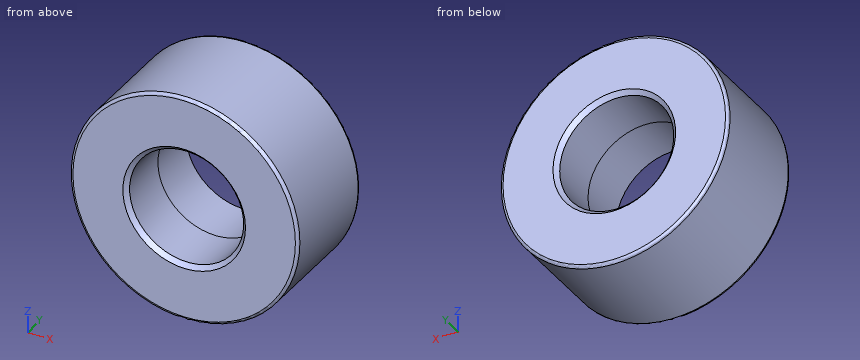
from build123d import *

# Parameters (mm, degrees)
SKETCH1_R                = 4
SKETCH1_R_2              = 2
BOSS_EXTRUDE1_DEPTH      = 1.875
BOSS_EXTRUDE1_DEPTH_BACK = 1.875
FILLET1_R                = 0.1
CHAMFER4_SIZE            = 0.15


with BuildPart() as part:
    # Sketch1 → Boss-Extrude1 (new body, two sides)
    with BuildSketch(Plane(origin=(0, 0, 0), x_dir=(1, 0, 0), z_dir=(0, 1, 0))) as boss_extrude1_sk:
        Circle(SKETCH1_R)
        Circle(SKETCH1_R_2, mode=Mode.SUBTRACT)
    extrude(amount=BOSS_EXTRUDE1_DEPTH)
    extrude(boss_extrude1_sk.sketch, amount=-BOSS_EXTRUDE1_DEPTH_BACK)

    # Fillet1
    fillet1_edges = [part.edges().sort_by_distance(p)[0] for p in [
        (-4, -1.875, 0),
        (-4, 1.875, 0),
    ]]
    fillet(fillet1_edges, radius=FILLET1_R)

    # Chamfer4
    chamfer4_edges = [part.edges().sort_by_distance(p)[0] for p in [
        (-2, -1.875, 0),
        (-2, 1.875, 0),
    ]]
    chamfer(chamfer4_edges, length=CHAMFER4_SIZE)


solid = part.part
Design review of the part built by this model. Coordinates are the model's own, in mm. Give positions to 0.01 mm unless a question says otherwise; leave off trailing zeros. Write each loop counter-clockwise with the first axis right and the second up, starting at its lowest first coordinate (ties: lowest second). Pieces come first, ordered by that corner, then holes. Notation, with made-up numbers: M 32,48.25 L 40,48.25 A7 cw 40,52.25 Z; hole C -15.75,-7 d9. An arc over 180 degrees is marked long. Return JSON: item names as keys, results as strings. Group by question number.
Item 1: Clearance check with a flat-ended pin moving along its axis: pin 1 Ø1.5 at (x, y) = (2.5, -1) entering from -Z. State where the tip first meets the part, or that it passes through.
Item 2: Wall thickness on line 1 along Z through (x, y) = (0, -0.8); line 2 along X through (y, z) = (-1.2, -0.75): over which ranges is each line inside the solid? List them lowest first.
Item 3: Take a section at A-A (x = 0). Give the boundary of the cut face in (y, z) (3 decimals), plus the area to 3 significant figures.
Item 4: Take a section at B-B (z = 0). Give the boundary of the cut face in (x, y) (3 decimals).
Item 5: Take a section at C-C (y = -0.3). Give the boundary of the cut face in (x, z).
Return value:
{
 "1": {"pin 1": "stops at z = -3.6"},
 "2": {"line 1": "z = -4 to -2, 2 to 4", "line 2": "x = -3.93 to -1.85, 1.85 to 3.93"},
 "3": {"outline": "M -1.875,-3.9 A0.1 ccw -1.775,-4 L 1.775,-4 A0.1 ccw 1.875,-3.9 L 1.875,-2.15 L 1.725,-2 L -1.725,-2 L -1.875,-2.15 Z; M -1.875,2.15 L -1.725,2 L 1.725,2 L 1.875,2.15 L 1.875,3.9 A0.1 ccw 1.775,4 L -1.775,4 A0.1 ccw -1.875,3.9 Z", "area": "14.9 mm2"},
 "4": {"outline": "M -4,-1.775 A0.1 ccw -3.9,-1.875 L -2.15,-1.875 L -2,-1.725 L -2,1.725 L -2.15,1.875 L -3.9,1.875 A0.1 ccw -4,1.775 Z; M 2,-1.725 L 2.15,-1.875 L 3.9,-1.875 A0.1 ccw 4,-1.775 L 4,1.775 A0.1 ccw 3.9,1.875 L 2.15,1.875 L 2,1.725 Z"},
 "5": {"outline": "C 0,0 d8; hole C 0,0 d4"}
}
